from build123d import *

# Parameters (mm, degrees)
BASE_EXTRUSION_DEPTH    = 36
BOSS_EXTRU_3_DEPTH      = 28
ESQUISSE6_R             = 4
ENL_V_MAT_EXTRU_2_DEPTH = 10


with BuildPart() as part:
    # Esquisse1 → Base-Extrusion (new body)
    with BuildSketch(Plane(origin=(0, 0, 0), x_dir=(0, 0, -1), z_dir=(1, 0, 0))):
        Polygon((0, 0), (0, 50), (18.5, 50), (18.5, 71), (63.5, 71), (63.5, 50), (82, 50), (82, 0), (54, 0), (54, 2), (57, 3.5), (57, 5), (22, 5), (22, 3.5), (25, 2), (25, 0), align=None)
    extrude(amount=BASE_EXTRUSION_DEPTH)

    # Esquisse5 → Boss.-Extru.3 (add)
    with BuildSketch(Plane(origin=(3, 0, 0), x_dir=(0, 0, -1), z_dir=(1, 0, 0))):
        with BuildLine():
            Line((26.042142261, 73.3389073), (17.839623353, 80.689282216))
            Line((17.839623353, 80.689282216), (20.510768328, 83.670098489))
            Line((20.510768328, 83.670098489), (29.512578974, 75.603468724))
            ThreePointArc((29.512578974, 75.603468724), (36.695776389, 74.476857579), (40, 68))
            Line((40, 68), (24, 68))
            ThreePointArc((24, 68), (24.527956708, 70.858070861), (26.042142261, 73.3389073))
        make_face()
    extrude(amount=BOSS_EXTRU_3_DEPTH)

    # Esquisse6 → Enlèv. mat.-Extru.2 (cut)
    with BuildSketch(Plane(origin=(0, 50, 0), x_dir=(-1, 0, 0), z_dir=(0, 1, 0))):
        with Locations(Location((-9, -8, 0), (0, 0, 90))):
            Circle(ESQUISSE6_R)
        with Locations(Location((-27, -8, 0), (0, 0, 90))):
            Circle(ESQUISSE6_R)
        with Locations((-45, -8)):
            Circle(ESQUISSE6_R)
        with Locations((-63, -8)):
            Circle(ESQUISSE6_R)
        with Locations(Location((-9, -74, 0), (0, 0, 90))):
            Circle(ESQUISSE6_R)
        with Locations(Location((-27, -74, 0), (0, 0, 90))):
            Circle(ESQUISSE6_R)
        with Locations((-45, -74)):
            Circle(ESQUISSE6_R)
        with Locations((-63, -74)):
            Circle(ESQUISSE6_R)
    extrude(amount=-ENL_V_MAT_EXTRU_2_DEPTH, mode=Mode.SUBTRACT)


solid = part.part
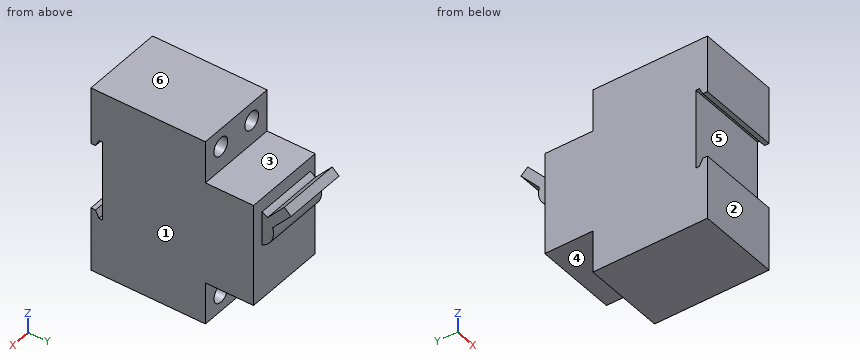
Source: CAD feature listing. Evaluate the final solid. Frame: model axes, mm. Face numbers are marked on the shaded views. A direction names the side the tool comes from. Give positions to 0.01 mm unless a question says otherwise; leave off trailing zeros. Write each loop counter-clockwise with the first axis right and the second up, starting at its lowest first coordinate (ties: lowest second). Pieces come first, ordered by that corner, then holes. Notation, with made-up numbers: (28, -9) -> (78, -9) arc R22 cw to (78, 3) -> close; hole circle Ø7 at (4, -0.75). An arc over 180 degrees is marked (long way). Return JSON: item names as keys, results as strings. Group by question number.
1. Section D-D, the plane y = 53. Output: boundary loops of the cut face in (x, z).
2. Section A-A, the plane y = 42. Output: boundary loops of the cut face in (x, z).
3. Pin query (flat end, axial travel): pin 1 Ø1.5 at (x, z) = (15, -73) entering from +Y; pin 2 Ø2 at (x, y) = (25.5, 62.5) entering from -Z; pin 3 Ø11 at (x, z) = (19, -52) entering from +Y; pin 4 Ø12 at (y, z) = (73, -72.5) entering from +X. Return the tip coordinate at first contact, or that it passes through.
4. Access query for the marked faces 4, 5 and 6. Directions: +Z, -Z, +X, -X, +Y, -Y. A direction counts if a zero-diameter tool reaches every point of the face in a straight line with its end or side. Return the directions, or none.
5. Mould query, pull axis Y, two halves, no side actions, for the marked faces 1, 2 and 3. Classes: +Y half, -Y half, draft (parallel to the pull), parting line (faces both ways), or undercut.
6. Section B-B, the plane z = -8. Output: boundary loops of the cut face in (x, y).
7. Material intervals for line 1 (X direction, y = 43.25, z = -74); line 2 (Z direction, x = 19, y = 4.5); line 3 (Y direction, x = 27, z = -11), sorted ascending. Write a range as from..to.
Determined:
{
 "1": {"outline": "(0, -63.5) -> (36, -63.5) -> (36, -18.5) -> (0, -18.5) -> close"},
 "2": {"outline": "(0, -82) -> (36, -82) -> (36, 0) -> (0, 0) -> close; hole circle Ø8 at (9, -74); hole circle Ø8 at (9, -8); hole circle Ø8 at (27, -74); hole circle Ø8 at (27, -8)"},
 "3": {"pin 1": "stops at y = 50", "pin 2": "stops at z = -63.5", "pin 3": "stops at y = 71", "pin 4": "passes through"},
 "4": {"face 4": "-Z, +X, -X, +Y", "face 5": "+X, -X", "face 6": "+Z, +X, -X, +Y, -Y"},
 "5": {"face 1": "draft", "face 2": "-Y half", "face 3": "undercut"},
 "6": {"outline": "(0, 0) -> (36, 0) -> (36, 50) -> (31, 50) -> (31, 40) -> (23, 40) -> (23, 50) -> (13, 50) -> (13, 40) -> (5, 40) -> (5, 50) -> (0, 50) -> close"},
 "7": {"line 1": "x = 0..5, 13..23, 31..36", "line 2": "z = -82..-57, -22..0", "line 3": "y = 0..40"}
}
